Source: CAD feature listing. Evaluate the final solid. Frame: model axes, mm. A direction names the side the tool comes from. Give positions to 0.01 mm unless a question says otherwise; leave off trailing zeros. Order: outer loops, then holes, each group sorted by start corner. A loop starts at its lowest first (then second) coordinate and runs counter-clockwise, first axis right, second up. Notation, with made-up numbers: (21.25, -35.5) - (26.25, -35.5) arc R18 cw to (26.25, -21.5) - close; hole circle Ø1 at (58, 22). An arc over 180 degrees is marked (long way). Use CSV: the item, a comma, the result in double quotes.
Autodesk Inventor part; units mm, degrees
ref_plane "Work Plane3" through (50, 2.5, 0) normal (-0.932, 0.3624, 0.0121) x (-0.3624, -0.932, 0)
ref_plane "Work Plane4" through (-7.3973, -145.1144, 0) normal (0.7449, -0.6672, 0) x (0.6672, 0.7449, 0)
ref_plane "YZ Plane" through (0, 0, 0) normal (1, 0, 0) x (0, 1, 0)
sketch "Sketch1" plane through (0, 0, 0) normal (0, 0, 1) x (1, 0, 0)
  line L0 (0, 0) -> (50, 0)
  line L1 (50, 0) -> (50, 5)
  line L2 (50, 5) -> (0, 5)
  line L3 (0, 5) -> (0, 0)
  dimension "d0" = 50
  dimension "d1" = 5
extrude "Extrusion1" add sketch "Sketch1" along normal blind 75
sketch "Sketch2" plane through (0, 0, 0) normal (-1, 0, 0) x (0, 0, 1)
  circle A0 centre (47.5, 2.5) radius 1
  circle A1 centre (27.5, 2.5) radius 1
  line L0 (0, 5) -> (0, 0)
  line L1 (0, 0) -> (75, 0)
  dimension "d4" = 2
  dimension "d5" = 2
  dimension "d6" = 27.5
  dimension "d7" = 20
  dimension "d8" = 2.5
extrude "Extrusion2" cut sketch "Sketch2" against normal blind 10
thread "Thread1"
thread "Thread2"
sketch "Sketch6" plane through (0, 0, 0) normal (0, 0, 1) x (1, 0, 0)
  circle A0 centre (-175, 5) radius 225 construction
  line L0 (-7.3973, 5.2329) -> (-7.3973, -145.1144) construction
  line L1 (-176.0104, 5) -> (50, 5) construction
  circle A1 centre (-175, 5) radius 220 construction
  arc A2 (-7.3973, -145.1144) -> (50, 5) centre (-175, 5) ccw
  line L2 (-7.3973, -145.1144) -> (-11.1218, -141.7785)
  arc A3 (-11.1218, -141.7785) -> (45, 5) centre (-175, 5) ccw
  line L3 (0, 5) -> (50, 5)
  line L4 (45, 5) -> (50, 5)
  point P0 (0, 5)
  dimension "d36" = 450
  dimension "d38" = 5
  dimension "d39" = 5
  dimension "d69" = 150.1144
extrude "Extrusion5" add sketch "Sketch6" along normal blind 75
ref_plane "Work Plane3" through (50, 2.5, 0) normal (-0.932, 0.3624, 0.0121) x (-0.3624, -0.932, 0)
sketch "Sketch7" plane through (50, 2.5, 0) normal (-0.932, 0.3624, 0.0121) x (-0.3624, -0.932, 0)
  circle A0 centre (27.1699, 27.4836) radius 3
  circle A1 centre (27.1699, 47.4836) radius 3
  line L0 (-2.3301, -0.0109) -> (-2.3301, 74.9836)
  circle A2 centre (37.1699, 27.4836) radius 3
  circle A3 centre (37.1699, 47.4836) radius 3
  point P0 (20.4501, -0.552)
  dimension "d42" = 6
  dimension "d43" = 6
  dimension "d44" = 29.5
  dimension "d46" = 20
  dimension "d47" = 27.5
  dimension "d48" = 6
  dimension "d49" = 6
  dimension "d50" = 10
extrude "Extrusion6" cut sketch "Sketch7" along normal through all both and the other way through all
sketch "Sketch8" plane through (0, 5, 0) normal (0, 1, 0) x (1, 0, 0)
  line L0 (5, -65) -> (45, -65)
  line L1 (45, -65) -> (45, -63)
  line L2 (45, -63) -> (5, -63)
  line L3 (5, -63) -> (5, -65)
  line L4 (50, 0) -> (0, 0)
  line L5 (0, 0) -> (0, -75)
  line L6 (50, -75) -> (0, -75)
  line L7 (50, 0) -> (50, -75)
  line L8 (45, -58) -> (5, -58)
  line L9 (5, -58) -> (5, -60)
  line L10 (5, -60) -> (45, -60)
  line L11 (45, -60) -> (45, -58)
  line L12 (45, -53) -> (5, -53)
  line L13 (5, -53) -> (5, -55)
  line L14 (5, -55) -> (45, -55)
  line L15 (45, -55) -> (45, -53)
  dimension "d56" = 40
  dimension "d57" = 2
  dimension "d58" = 5
  dimension "d59" = 10
  dimension "d62" = 5
extrude "Extrusion7" cut sketch "Sketch8" against normal blind 5 contours L3 L2 L1 L0 | L11 L10 L9 L8 | L15 L14 L13 L12
ref_plane "Work Plane4" through (-7.3973, -145.1144, 0) normal (0.7449, -0.6672, 0) x (0.6672, 0.7449, 0)
sketch "Sketch9" plane through (-7.3973, -145.1144, 0) normal (0.7449, -0.6672, 0) x (0.6672, 0.7449, 0)
  circle A0 centre (6, 27.5) radius 3
  circle A1 centre (6, 47.5) radius 3
  line L0 (146.3528, 75) -> (0, 75)
  line L1 (0, 0) -> (0, 75)
  point P0 (113.0311, 0)
  dimension "d70" = 6
  dimension "d71" = 6
  dimension "d72" = 27.5
  dimension "d73" = 20
  dimension "d74" = 6
extrude "Extrusion8" cut sketch "Sketch9" along normal through all both and the other way through all
sketch "Sketch10" plane through (0, 0, 0) normal (0, 0, -1) x (-1, 0, 0)
  circle A0 centre (175, 5) radius 225
  circle A1 centre (175, 5) radius 230
  point P0 (-49.9444, 0)
  point P1 (-50, 5)
  dimension "d77" = 450
  dimension "d78" = 5
extrude "Extrusion9" cut sketch "Sketch10" against normal through all
properties part number "CW002" material "ABS Plastic"
Item 1: Set-up query: faces 4 (the flat face through (0, 3, 37)), 5 (the flat face through (25, 3, 53)), 6 (the flat face through (22, 0, 37)). Return all of +Z, -Z, +X, -X, +Y, -Y with unobstructed straight access to the full face (end or side cutting, diameter ignored); none if empty.
Filled in:
face 4,"+Z, -Z, -X, +Y"
face 5,"+Y"
face 6,"+Z, -Z, -X"
Item 2: Material intervals for line 1 (Y direction, x = 8, z = 47.5); line 2 (Y direction, x = 5, z = 47.5); line 3 (Z direction, x = 7, y = 2), sorted ascending. Write a range as from..to.
Filled in:
line 1,"y = -125.9..-117.11, 0..1.5, 3.5..5"
line 2,"y = -130..-121.49, 0..1.5, 3.5..5"
line 3,"z = 0..26.63, 28.37..46.63, 48.37..53, 55..58, 60..63, 65..75"
Item 3: Section D-D on x = 39.5. Return the cut outline in (y, z), then the cut area to 3 significant figures.
Filled in:
outline,"(-62.93, 0) - (-43.89, 0) - (-43.89, 75) - (-62.93, 75) - close; (0, 0) - (5, 0) - (5, 53) - (0, 53) - close; (0, 55) - (5, 55) - (5, 58) - (0, 58) - close; (0, 60) - (5, 60) - (5, 63) - (0, 63) - close; (0, 65) - (5, 65) - (5, 75) - (0, 75) - close"
area,"1,770 mm2"
Item 4: Section B-B on x = 18.5. Return the cut outline in (y, z), then the cut area to 3 significant figures.
Filled in:
outline,"(-109.82, 0) - (-99.68, 0) - (-99.68, 75) - (-109.82, 75) - close; (0, 0) - (5, 0) - (5, 53) - (0, 53) - close; (0, 55) - (5, 55) - (5, 58) - (0, 58) - close; (0, 60) - (5, 60) - (5, 63) - (0, 63) - close; (0, 65) - (5, 65) - (5, 75) - (0, 75) - close"
area,"1,110 mm2"
Item 5: Mould query, pull axis X, two halves, no side actions, for faces 1 (the flat face through (37, -59, 0)), 2 (the cylindrical face through (34.663, -76.649, 36.975)), 3 (the cylindrical face through (-6.78, -140.58, 49.53)). Classes: released by +X, released by -X, zero draft, split by the parting line, or undercut.
Filled in:
face 1,"zero draft"
face 2,"released by +X"
face 3,"undercut"
Item 6: Section C-C on y = -80.5. Return the cut outline in (x, z).
Filled in:
outline,"(27.71, 0) - (33.12, 0) - (33.12, 75) - (27.71, 75) - close"
Item 7: First-contact query: pin 1 (8 mm diameter, centred on y = -105.5, z = 45.5, fed in from -X); pin 2 (1 mm diameter, centred on x = 6.5, y = -117, fed in from -Z); pin 3 (5.5 mm diameter, centred on y = 3, z = 26, fed in from -X); pin 4 (8 mm diameter, centred on y = -43, z = 57.5, fed in from +X). Flat tips, straight axial feed; report the tip coordinate or a pass-through.
Filled in:
pin 1,"stops at x = 12.86"
pin 2,"passes through"
pin 3,"stops at x = 0"
pin 4,"stops at x = 45.66"
Item 8: Section A-A on x = 2. Return the cut outline in (y, z).
Filled in:
outline,"(-133.91, 0) - (-125.66, 0) - (-125.66, 75) - (-133.91, 75) - close; (0, 0) - (5, 0) - (5, 75) - (0, 75) - close; hole circle Ø2 at (2.5, 27.5); hole circle Ø2 at (2.5, 47.5)"
